from build123d import *

# Parameters (mm, degrees)
IZIM1_W                     = 17
IZIM1_H                     = 2.55
IZIM4_R                     = 2.575
Y_KSEKLIK_EKSTR_ZYON1_DEPTH = 0.6
IZIM5_R                     = 3.175
Y_KSEKLIK_EKSTR_ZYON2_DEPTH = 3.4
IZIM7_R                     = 2.575
Y_KSEKLIK_EKSTR_ZYON4_DEPTH = 0.6
Y_KSEKLIK_EKSTR_ZYON5_START = 3.4
IZIM8_R                     = 3.175
Y_KSEKLIK_EKSTR_ZYON5_DEPTH = 3.4
IZIM9_R                     = 1.65
KES_EKSTR_ZYON1_DEPTH       = 100
PAH1_SIZE                   = 0.1


# Read off the part's stored shape, not the designer's step: Draft2, Draft3
with BuildPart() as part:
    # Çizim1 → Döndür3 (revolve)
    with BuildSketch(Plane(origin=(0, 0, 0), x_dir=(0, 0, -1), z_dir=(1, 0, 0)), mode=Mode.PRIVATE) as d_nd_r3_sk:
        with Locations((0, -1.275)):
            Rectangle(IZIM1_W, IZIM1_H)
    revolve(d_nd_r3_sk.sketch.rotate(Axis((0, 0, 15.544933078), (0, 0, -1)), 270), axis=Axis((0, 0, 15.544933078), (0, 0, -1)))

    # Çizim4 → Yükseklik-Ekstrüzyon1 (add)
    with BuildSketch(Plane(origin=(0, 0, -8.5), x_dir=(-1, 0, 0), z_dir=(0, 0, -1))):
        Circle(IZIM4_R)
    extrude(amount=Y_KSEKLIK_EKSTR_ZYON1_DEPTH)

    # Çizim5 → Yükseklik-Ekstrüzyon2 (add)
    with BuildSketch(Plane(origin=(0, 0, -9.1), x_dir=(-1, 0, 0), z_dir=(0, 0, -1))):
        Circle(IZIM5_R)
    extrude(amount=Y_KSEKLIK_EKSTR_ZYON2_DEPTH)

    # Draft2 outline → Draft2 (revolve)
    with BuildSketch(Plane.XZ):
        Polygon((3.175, -9.003459779), (2.575, -8.5), (2.575, -9.1), (3.175, -9.1), align=None)
    revolve(axis=Axis((0, 0, 0), (0, 0, 1)))

    # Çizim7 → Yükseklik-Ekstrüzyon4 (add)
    with BuildSketch(Plane.XY.offset(8.5)):
        Circle(IZIM7_R)
    extrude(amount=Y_KSEKLIK_EKSTR_ZYON4_DEPTH)

    # Çizim8 → Yükseklik-Ekstrüzyon5 (add)
    with BuildSketch(Plane.XY.offset(9.1).offset(Y_KSEKLIK_EKSTR_ZYON5_START)):
        with Locations(Location((0, 0, 0), (0, 0, 180))):
            Circle(IZIM8_R)
    extrude(amount=-Y_KSEKLIK_EKSTR_ZYON5_DEPTH)

    # Draft3 outline → Draft3 (revolve)
    with BuildSketch(Plane.XZ):
        Polygon((2.575, 8.5), (3.175, 9.003459779), (3.175, 9.1), (2.575, 9.1), align=None)
    revolve(axis=Axis((0, 0, 0), (0, 0, 1)))

    # Çizim9 → Kes-Ekstrüzyon1 (cut)
    with BuildSketch(Plane.XY.offset(12.5)):
        Circle(IZIM9_R)
    extrude(amount=-KES_EKSTR_ZYON1_DEPTH, mode=Mode.SUBTRACT)

    # Pah1
    pah1_edges = [part.edges().sort_by_distance(p)[0] for p in [
        (3.175, 0, -12.5),
        (3.175, 0, 12.5),
    ]]
    chamfer(pah1_edges, length=PAH1_SIZE)


solid = part.part
Model file for the job. Use its own axes, mm. Round coordinates to 2 decimals unless told otherwise and drop trailing zeros. Loops run counter-clockwise (first coordinate to the right, second up) from the corner with the lowest first, then second, coordinate; pieces in that order, holes last.
1. Band-saw the part on D-D, the plane z = 10.25. List the corners of the cut face in (x, y) (3 decimals), and give its area (3 significant figures).
Check values:
outline: circle Ø6.35 at (0, 0); hole circle Ø3.3 at (0, 0)
area: 23.1 mm2
2. Band-saw the part on A-A, the plane x = 0. List the corners of the cut face in (y, z) (3 decimals), and give its area (3 significant figures).
Check values:
outline: (-3.175, -12.4) - (-3.075, -12.5) - (-1.65, -12.5) - (-1.65, 12.5) - (-3.075, 12.5) - (-3.175, 12.4) - (-3.175, 9.003) - (-2.575, 8.5) - (-2.55, 8.5) - (-2.55, -8.5) - (-2.575, -8.5) - (-3.175, -9.003) - close; (1.65, -12.5) - (3.075, -12.5) - (3.175, -12.4) - (3.175, -9.003) - (2.575, -8.5) - (2.55, -8.5) - (2.55, 8.5) - (2.575, 8.5) - (3.175, 9.003) - (3.175, 12.4) - (3.075, 12.5) - (1.65, 12.5) - close
area: 54.4 mm2
3. Drop flat-ended pins along their axis: P1, Ø1.5, axis at y = 0.5, z = -5.5, coming from the -X side; P2, Ø1.5, axis at x = 0.5, z = -7, coming from the -Y side. Give the stop position or say it passes through.
Check values:
P1: stops at x = -2.55
P2: stops at y = -2.55
4. Mould opens along X. For faces 1 (the flat face through (-1.3, 1.3, 12.5)), 2 (the cylindrical face through (-1.216, 1.115, 0.175)), 3 (the cylindrical face through (2.43, -0.77, -0.12)) say: +X half, -X half, draft (parallel to the pull), parting line (faces both ways), or undercut.
Check values:
face 1: draft
face 2: undercut
face 3: parting line
5. Wall check: probe 1 along Y at (x, z) = (0, 2.75); probe 2 along Y at (x, z) = (0, 11.25) (3 decimals); probe 3 along X at (y, z) = (0.5, 7.75). Give the ranges that are in metal, low to high.
Check values:
probe 1: y = -2.55 to -1.65, 1.65 to 2.55
probe 2: y = -3.175 to -1.65, 1.65 to 3.175
probe 3: x = -2.5 to -1.57, 1.57 to 2.5
6. Band-saw the part on C-C, the plane z = -5. List the corners of the cut face in (x, y), and give its area (3 significant figures).
Check values:
outline: circle Ø5.1 at (0, 0); hole circle Ø3.3 at (0, 0)
area: 11.9 mm2
